Autodesk Inventor part; units mm, degrees
ref_plane "Plano de correa" through (0, 146.5, 10) normal (0, 0, 1) x (1, 0, 0)
ref_plane "YZ Plane" through (0, 0, 0) normal (1, 0, 0) x (0, 1, 0)
ref_plane "XZ Plane" through (0, 0, 0) normal (0, 1, 0) x (-1, 0, 0)
sketch "Boceto principal" plane through (0, 0, 0) normal (1, 0, 0) x (0, 1, 0)
  line L0 (0, 20) -> (160.3, 20)
  line L1 (160.3, 20) -> (160.3, 16.356)
  line L2 (160.3, 16.356) -> (146.5, 12.137)
  line L3 (146.5, 12.137) -> (146.5, 7.863)
  line L4 (146.5, 7.863) -> (160.3, 3.644)
  line L5 (160.3, 3.644) -> (160.3, 0)
  line L6 (160.3, 0) -> (0, 0)
  line L7 (157.5, 15.5) -> (157.5, 4.5) construction
  line L8 (146.5, 10) -> (157.5, 10) construction
  line L9 (160.3, 16.356) -> (160.3, 3.644)
  line L10 (0, -4) -> (0, 24)
  line L11 (0, 0) -> (0, 20)
  dimension "d0" = 11
  dimension "d1" = 34
  dimension "d2" = 2.8
  dimension "d6" = 20
  dimension "d21" = 315
  dimension "d25" = 13.8
  dimension "d27" = 10
ref_plane "Plano de correa" through (0, 146.5, 10) normal (0, 0, 1) x (1, 0, 0)
revolve "Cuerpo" add sketch "Boceto principal" angle 360 about axis through (0, 0, -10) along (0, 0, 1)
revolve "Para ranuras" cut sketch "Boceto principal" angle 360 about axis through (0, 0, -10) along (0, 0, 1) contours L9 L4 L3 L2
fillet "Empalme externo" [suppressed]
fillet "Empalme interno" [suppressed]
pattern_of_one "Patrón para ranuras"
equation "\"d0\" = da_Bw"
equation "\"d1\" = da_Alfa"
equation "\"d2\" = da_c"
equation "\"d21\" = da_Dw"
equation "\"d25\" = da_Hd"
equation "\"d27\" = da_Se"
equation "\"da_r1\" = 0"
equation "\"da_r2\" = 0"
equation "\"d18\" = da_Sg"
equation "\"da_Bw\" = 11"
equation "\"da_Alfa\" = 34deg"
equation "\"da_c\" = 2.8"
equation "\"da_Dw\" = 315"
equation "\"da_Hd\" = 13.8"
equation "\"da_Se\" = 10"
equation "\"da_Sg\" = 15"
properties part number "Polea ranurada2" material "Steel"
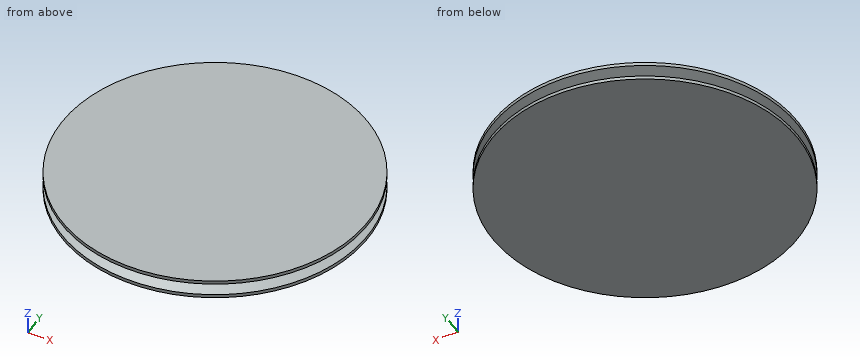
Work out the finished part from the listing and answer in its coordinate system (mm). Round coordinates to 2 decimals unless told otherwise and drop trailing zeros. Write each loop counter-clockwise with the first axis right and the second up, starting at its lowest first coordinate (ties: lowest second). Pieces come first, ordered by that corner, then holes. Notation, with made-up numbers: (46.5, 21) -> (89.5, 21) arc R31 cw to (89.5, 52) -> close; hole circle Ø11 at (39.5, 86). An arc over 180 degrees is marked (long way). Write each question's results on one line, items separated by ' | '.
Q1. Flat-ended cylindrical pins translate along their axes: P1, Ø4, axis at x = 87.5, z = 4.5, coming from the +Y side; P2, Ø8, axis at x = -59, z = 5.5, coming from the +Y side; P3, Ø12, axis at y = -18, z = 4, coming from the -X side. Find the tip coordinate at first contact, or state that the pin passes through.
Data:
P1: y = 135.47 | P2: y = 150.4 | P3: x = -159.85
Q2. Section A-A, the plane y = 0 is taken. Write down the section's boundary in (x, z), then the cut area to 3 significant figures.
Data:
outline: (-160.3, 0) -> (160.3, 0) -> (160.3, 3.64) -> (146.5, 7.86) -> (146.5, 12.14) -> (160.3, 16.36) -> (160.3, 20) -> (-160.3, 20) -> (-160.3, 16.36) -> (-146.5, 12.14) -> (-146.5, 7.86) -> (-160.3, 3.64) -> close | area: 6,180 mm^2
Q3. Straight lines are drawn through the part: line 1 along Y through (x, z) = (34.5, 1.5); line 2 along X through (y, z) = (19.5, 18.75); line 3 along Y through (x, z) = (-125.5, 18). For each, find the intervals that lie inside material, in ascending order. Write a range as [from, to].
Data:
line 1: [-156.54, 156.54] | line 2: [-159.11, 159.11] | line 3: [-99.73, 99.73]
